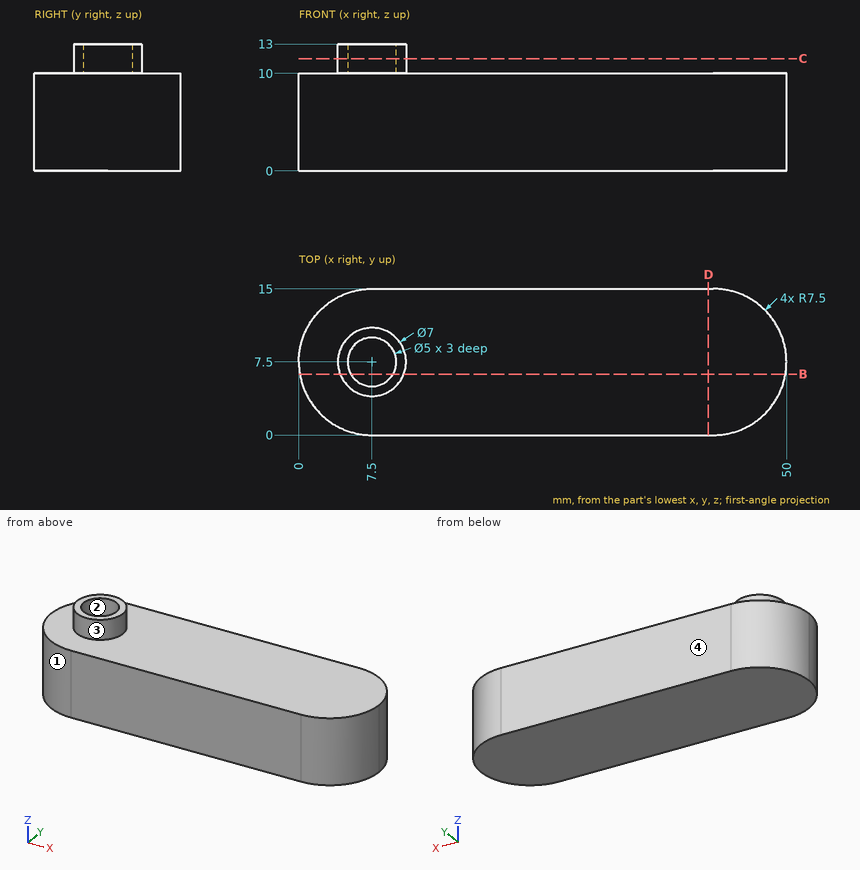
Verification items for this drawing (mm, ordinates from the low corner). Round coordinates to 2 decimals unless told otherwise and drop trailing zeros. Loops run counter-clockwise (first coordinate to the right, second up) from the corner with the lowest first, then second, coordinate; pieces in that order, holes last. Notation, with made-up numbers: (29, -31) - (55, -31) arc R32 ccw to (55, 7) - close; hole circle Ø1 at (62.25, 9). An arc over 180 degrees is marked (long way). Answer as CSV lines item,"result". Start each with the question number.
Item 1: Section check C-C (z = 11.5). Record the boundary of the cut face in (x, y).
Item 2: Section check D-D (x = 42). Record the boundary of the cut face in (y, z), and give its area (3 significant figures).
Item 3: Section check B-B (y = 6.25). Record the boundary of the cut face in (x, z) (3 decimals).
Item 4: Scan lines: line 1 (Y direction, x = 7.5, z = 10.8); line 2 (Z direction, x = 14, y = 6.75); line 3 (X direction, y = 4.75, z = 12) (1 decimal). Record each from-to range of solid material in increasing order. Write a range as [from, to].
Item 5: Release check for a two-part mould opening along X. For the marked faces 1, 2, 3 and 4 record: +X half, -X half, draft (parallel to the pull), parting line (faces both ways), or undercut.
Item 6: Depth check by flat-ended pin: P1, Ø4, axis at y = 11, z = 5.5, coming from the -X side; P2, Ø2.5, axis at x = 7, y = 6.5, coming from the +Z side; P3, Ø1.5, axis at y = 3.5, z = 6.5, coming from the +X side. Enter the tip coordinate at first touch or a pass-through.
Report:
1,outline,"circle Ø7 at (7.5, 7.5); hole circle Ø5 at (7.5, 7.5)"
2,outline,"(0, 0) - (15, 0) - (15, 10) - (0, 10) - close"
2,area,"150 mm2"
3,outline,"(0.105, 0) - (49.895, 0) - (49.895, 10) - (10.769, 10) - (10.769, 13) - (9.665, 13) - (9.665, 10) - (5.335, 10) - (5.335, 13) - (4.231, 13) - (4.231, 10) - (0.105, 10) - close"
4,line 1,"y = [4, 5], [10, 11]"
4,line 2,"z = [0, 10]"
4,line 3,"x = [5.3, 9.7]"
5,face 1,"-X half"
5,face 2,"undercut"
5,face 3,"parting line"
5,face 4,"draft"
6,P1,"stops at x = 0.15"
6,P2,"stops at z = 10"
6,P3,"stops at x = 49.26"
